Geometry: final body of the model. Coordinates: model frame, mm. A direction names the side the tool comes from. Coordinates: 2 decimals unless noted, no trailing zeros. Write each loop counter-clockwise with the first axis right and the second up, starting at its lowest first coordinate (ties: lowest second). Pieces come first, ordered by that corner, then holes. Notation, with made-up numbers: (-18.75, -2.75) -> (29.25, -2.75) arc R16 cw to (29.25, 8.25) -> close; hole circle Ø2 at (59.5, 1). An arc over 180 degrees is marked (long way). Answer as a JSON object with one key per item and string values. Group by question number.
```python
from build123d import *

# Parameters (mm, degrees)
SKETCH_1_W          = 3.5
SKETCH_1_H          = 12.1
EXTRUDE_1_DEPTH     = 13.2
SKETCH_2_W          = 0.330714911
SKETCH_2_H          = 1.671791026
CUT_EXTRUDE_1_DEPTH = 13.2
SKETCH_8_W          = 0.257824974
SKETCH_8_H          = 3.133485684
CUT_EXTRUDE_4_DEPTH = 2
SKETCH_4_R          = 1.25
CUT_EXTRUDE_2_DEPTH = 5
CUT_EXTRUDE_3_DEPTH = 0.5
SKETCH_6_W          = 0.8
SKETCH_6_H          = 0.4
EXTRUDE_1424_DEPTH  = 4


with BuildPart() as part:
    # 草图1 → 凸台-拉伸1 (new body)
    with BuildSketch(Plane(origin=(0, 0, 0), x_dir=(1, 0, 0), z_dir=(0, 1, 0))):
        Rectangle(SKETCH_1_W, SKETCH_1_H)
    extrude(amount=EXTRUDE_1_DEPTH)

    # 草图2 → 切除-拉伸1 (cut)
    with BuildSketch(Plane.ZY.offset(1.75)):
        with Locations((-5.884642545, 4.259492563)):
            Rectangle(SKETCH_2_W, SKETCH_2_H)
        Polygon((-4.4584027, 12.092198582), (-6.05, 9.129739953), (-6.05, 13.2), (-1.750507475, 13.2), (-2.117021791, 12.824491726), (-2.117021791, 12.39177305), (-1.750507475, 12.39177305), (-1.750507475, 9.747762053), (-3.260104827, 11.218439716), (-3.260104827, 12.092198582), align=None)
        Polygon((1.382978209, 13.2), (1.382978209, 10.565811036), (2.140809297, 11.977057019), (3.463073776, 11.977057019), (6.05, 7.365579196), (6.05, 13.2), align=None)
    extrude(amount=-CUT_EXTRUDE_1_DEPTH, mode=Mode.SUBTRACT)

    # 草图8 → 切除-拉伸4 (cut)
    with BuildSketch(Plane(origin=(0, 13.2, 0), x_dir=(1, 0, 0), z_dir=(0, 1, 0))):
        with Locations((1.621087513, 0.183764633)):
            Rectangle(SKETCH_8_W, SKETCH_8_H)
        with Locations((-1.621087513, 0.183764633)):
            Rectangle(SKETCH_8_W, SKETCH_8_H)
    extrude(amount=-CUT_EXTRUDE_4_DEPTH, mode=Mode.SUBTRACT)

    # 草图4 → 切除-拉伸2 (cut)
    with BuildSketch(Plane(origin=(0, 4.344588307, 7.744701971), x_dir=(1, 0, 0), z_dir=(0, 0.4892509225965462, 0.8721430701085852))):
        with Locations(Location((0, 5.619309483, 0), (0, 0, 270))):
            Circle(SKETCH_4_R)
    extrude(amount=-CUT_EXTRUDE_2_DEPTH, mode=Mode.SUBTRACT)

    # 草图5 → 切除-拉伸3 (cut)
    with BuildSketch(Plane(origin=(0, 13.2, 0), x_dir=(1, 0, 0), z_dir=(0, 1, 0))):
        Polygon((-2.244287714, 1.689705222), (-1.702195493, 2.211037938), (2.310317802, -1.381291481), (1.810052614, -1.94007117), align=None)
    extrude(amount=-CUT_EXTRUDE_3_DEPTH, mode=Mode.SUBTRACT)

    # 草图6 → Extrude 1424 (add)
    with BuildSketch(Plane.XZ):
        with Locations((0, 2.05)):
            Rectangle(SKETCH_6_W, SKETCH_6_H)
    extrude(amount=EXTRUDE_1424_DEPTH)


solid = part.part
```
Item 1: Section D-D on y = 4.5. Output: boundary loops of the cut face in (x, z).
Item 2: Contact query for flat-ended pins moving along their axis: pin 1 (1.5 mm diameter, centred on x = 0.5, z = 2.5, fed in from +Y); pin 2 (0.6 mm diameter, centred on y = 12.5, z = 0.5, fed in from -X); pin 3 (2 mm diameter, centred on x = 0.5, y = 10.5, fed in from -Z). Output: stop coordinate, or through.
Item 3: Section A-A on x = -0.8. Output: boundary loops of the cut face in (y, z), then the cut area to 3 significant figures.
Item 4: Set-up query: faces 1 (the flat face through (0, 11, -1.751)), 2 (the flat face through (0, 12.092, -4)), 3 (the flat face through (0, 12.7, 0)). Return all of +Z, -Z, +X, -X, +Y, -Y with unobstructed straight access to the full face (end or side cutting, diameter ignored); none if empty.
Item 5: Ray query, L1, parallel to X at y = 9.5, z = 4.25; L2, parallel to Y at x = -1.35, z = -1; L3, parallel to Y at x = 0.7, z = 0.5. Return the intervals inside material, ascending. Write a range as [from, to].
Item 6: Section C-C on y = -2.5. Output: boundary loops of the cut face in (x, z), then the cut area to 3 significant figures.
Item 7: Section B-B on z = -0.25. Output: boundary loops of the cut face in (x, y).
Item 8: Mould query, pull axis X, two halves, no side actions, for faces 4 (the flat face through (0.02, 6.81, 0.63)), 5 (the flat face through (0, 11.6, -3.26)), 6 (the flat face through (1.75, 6, 0)). Classes: +X half, -X half, draft (parallel to the pull), parting line (faces both ways), or undercut.
Answer sheet:
{
 "1": {"outline": "(-1.75, -5.72) -> (1.75, -5.72) -> (1.75, 6.05) -> (-1.75, 6.05) -> close"},
 "2": {"pin 1": "stops at y = 11.98", "pin 2": "stops at x = -1.49", "pin 3": "stops at z = -5.85"},
 "3": {"outline": "(0, -6.05) -> (3.42, -6.05) -> (3.42, -5.72) -> (5.1, -5.72) -> (5.1, -6.05) -> (9.13, -6.05) -> (12.09, -4.46) -> (12.09, -3.26) -> (11.22, -3.26) -> (9.75, -1.75) -> (12.39, -1.75) -> (12.39, -2.12) -> (12.82, -2.12) -> (13.2, -1.75) -> (13.2, -1.4) -> (12.7, -1.4) -> (12.7, -0.4) -> (13.2, -0.4) -> (13.2, 1.38) -> (10.57, 1.38) -> (11.98, 2.14) -> (11.98, 3.46) -> (10.08, 4.53) -> (7.64, 0.16) -> (5.96, 1.1) -> (8.41, 5.47) -> (7.37, 6.05) -> (0, 6.05) -> close", "area": "128 mm^2"},
 "4": {"face 1": "+X, -X", "face 2": "-Z, +X, -X, +Y", "face 3": "+Y"},
 "5": {"L1": "x = [-1.75, -1.1], [1.1, 1.75]", "L2": "y = [0, 12.7]", "L3": "y = [0, 7.04], [7.91, 12.7]"},
 "6": {"outline": "(-0.4, 1.85) -> (0.4, 1.85) -> (0.4, 2.25) -> (-0.4, 2.25) -> close", "area": "0.320 mm^2"},
 "7": {"outline": "(-1.75, 0) -> (1.75, 0) -> (1.75, 11.2) -> (1.49, 11.2) -> (1.49, 13.2) -> (0.49, 13.2) -> (0.49, 12.7) -> (-0.64, 12.7) -> (-0.64, 13.2) -> (-1.49, 13.2) -> (-1.49, 11.2) -> (-1.75, 11.2) -> close"},
 "8": {"face 4": "undercut", "face 5": "draft", "face 6": "+X half"}
}
